Model file for the job. Use its own axes, mm. A direction names the side the tool comes from. Give positions to 0.01 mm unless a question says otherwise; leave off trailing zeros. Order: outer loops, then holes, each group sorted by start corner. A loop starts at its lowest first (then second) coordinate and runs counter-clockwise, first axis right, second up. Notation, with made-up numbers: (69, 15.25) -> (82, 15.25) arc R15 ccw to (82, 21.25) -> close; hole circle Ø3 at (-15, 36). An arc over 180 degrees is marked (long way). Use CSV: the item, a comma, the result in double quotes. Start each with the question number.
1. Cut at A-A on y = 0. List the corners of the cut face in (x, z), then the cut area to 3 significant figures.
2. Wall check: line 1 (Z direction, x = 40, y = -10.75); line 2 (Y direction, x = 37, z = 2.5). Give the ranges that are in metal, low to high. Write a range as from..to.
3. Drop flat-ended pins along their axis: pin 1 (5 mm diameter, centred on x = 15, z = -2, fed in from -Y); pin 2 (12 mm diameter, centred on x = 44, z = 9.5, fed in from -Y); pin 3 (6 mm diameter, centred on x = -34.5, z = 7.5, fed in from +Y); pin 4 (1.9 mm diameter, centred on y = 2.5, z = 9.5, fed in from +X). Give the stop position or say it passes through.
4. Cut at D-D on y = -7. List the corners of the cut face in (x, z), then the cut area to 3 significant figures.
5. 3-axis set-ups, long thin cutter, end or side, ignore diameter. For faces 1 (the flat face through (38.1, 0, 9)), 2 (the flat face through (-63.5, 0.9, 11.3)), 3 (the flat face through (38.1, 0, -9)): which of +Z, -Z, +X, -X, +Y, -Y reach the whole face in a straight line?
6. Cut at C-C on x = -46.5. List the corners of the cut face in (y, z), then the cut area to 3 significant figures.
7. Cut at B-B on z = 0. List the corners of the cut face in (x, y), then the cut area to 3 significant figures.
```python
from build123d import *

# Parameters (mm, degrees)
F0_R     = 12.6365
F1_DEPTH = 63.5
F2_W     = 25.4
F2_H     = 6.2865
F3_DEPTH = 12.7
F4_W     = 25.4
F4_H     = 6.2865
F5_DEPTH = 12.7


with BuildPart() as f1:
    # F0 (on Right) → F1 (new body, symmetric)
    with BuildSketch(Plane.YZ):
        Circle(F0_R)
    extrude(amount=F1_DEPTH, both=True)

    # F2 (on Front) → F3 (cut, symmetric)
    with BuildSketch(Plane.XZ):
        with Locations((50.8, 9.49325)):
            Rectangle(F2_W, F2_H)
    extrude(amount=F3_DEPTH, both=True, mode=Mode.SUBTRACT)

    # F4 (on Front) → F5 (cut, symmetric)
    with BuildSketch(Plane.XZ):
        with Locations((50.8, -9.49325)):
            Rectangle(F4_W, F4_H)
    extrude(amount=F5_DEPTH, both=True, mode=Mode.SUBTRACT)

    # F6 (on Front) → F7 (revolve, cut)
    with BuildSketch(Plane.XZ):
        with BuildLine():
            Line((-69.85, -12.7), (-69.85, 12.7))
            ThreePointArc((-69.85, 12.7), (-82.55, 0), (-69.85, -12.7))
        make_face()
    revolve(axis=Axis((-69.85, 0, 0), (0, 0, -1)), mode=Mode.SUBTRACT)


solid = f1.part
```
Verdict:
1,outline,"(-63.5, -12.64) -> (38.1, -12.64) -> (38.1, -6.35) -> (63.5, -6.35) -> (63.5, 6.35) -> (38.1, 6.35) -> (38.1, 12.64) -> (-63.5, 12.64) -> (-63.5, 11) arc R12.7 cw to (-63.5, -11) -> close"
1,area,"2,790 mm^2"
2,line 1,"-6.35..6.35"
2,line 2,"-12.39..12.39"
3,pin 1,"y = -12.64"
3,pin 2,"y = -12.14"
3,pin 3,"y = 11.81"
3,pin 4,"x = 38.1"
4,outline,"(-63.5, -10.52) -> (38.1, -10.52) -> (38.1, -6.35) -> (63.5, -6.35) -> (63.5, 6.35) -> (38.1, 6.35) -> (38.1, 10.52) -> (-63.5, 10.52) -> (-63.5, 8.48) arc R10.6 cw to (-63.5, -8.48) -> close"
4,area,"2,410 mm^2"
5,face 1,"+Z, +X, +Y, -Y"
5,face 2,"+Z, -Z, -X, +Y, -Y"
5,face 3,"-Z, +X, +Y, -Y"
6,outline,"circle Ø25.27 at (0, 0)"
6,area,"502 mm^2"
7,outline,"(-63.5, -12.64) -> (63.5, -12.64) -> (63.5, 12.64) -> (-63.5, 12.64) -> (-63.5, 11) arc R12.7 cw to (-63.5, -11) -> close"
7,area,"3,110 mm^2"
